from build123d import *

# Parameters (mm, degrees)
SKETCH_1_R          = 1.8
EXTRUDE_1_DEPTH     = 6.4
SKETCH_7_R          = 3
CUT_EXTRUDE_1_DEPTH = 3.2
SKETCH_8_R          = 4
SKETCH_8_R_2        = 1.8
EXTRUDE_2_DEPTH     = 5
SKETCH_9_R          = 5.65
SKETCH_9_R_2        = 4
CUT_EXTRUDE_2_DEPTH = 2


with BuildPart() as part:
    # Эскиз1 → Бобышка-Вытянуть1 (new body)
    with BuildSketch(Plane(origin=(0, 0, 0), x_dir=(1, 0, 0), z_dir=(0, 1, 0))):
        with BuildLine():
            Line((-10, 0), (-8.31553819, 3.436118058))
            ThreePointArc((-8.31553819, 3.436118058), (-1.40535605, 7.805603403), (5.613555936, 3.613003503))
            Line((5.613555936, 3.613003503), (7.5, 0))
            Line((7.5, 0), (5.613555936, -3.613003503))
            ThreePointArc((5.613555936, -3.613003503), (-1.40535605, -7.805603403), (-8.31553819, -3.436118058))
            Line((-8.31553819, -3.436118058), (-10, 0))
        make_face()
        Circle(SKETCH_1_R, mode=Mode.SUBTRACT)
    extrude(amount=EXTRUDE_1_DEPTH)

    # Эскиз7 → Вырез-Вытянуть1 (cut)
    with BuildSketch(Plane(origin=(0, 6.4, 0), x_dir=(1, 0, 0), z_dir=(0, 1, 0))):
        Circle(SKETCH_7_R)
    extrude(amount=-CUT_EXTRUDE_1_DEPTH, mode=Mode.SUBTRACT)

    # Эскиз8 → Бобышка-Вытянуть2 (add)
    with BuildSketch(Plane.XZ):
        Circle(SKETCH_8_R)
        Circle(SKETCH_8_R_2, mode=Mode.SUBTRACT)
    extrude(amount=EXTRUDE_2_DEPTH)

    # Эскиз9 → Вырез-Вытянуть2 (cut)
    with BuildSketch(Plane.XZ):
        Circle(SKETCH_9_R)
        Circle(SKETCH_9_R_2, mode=Mode.SUBTRACT)
    extrude(amount=-CUT_EXTRUDE_2_DEPTH, mode=Mode.SUBTRACT)


solid = part.part
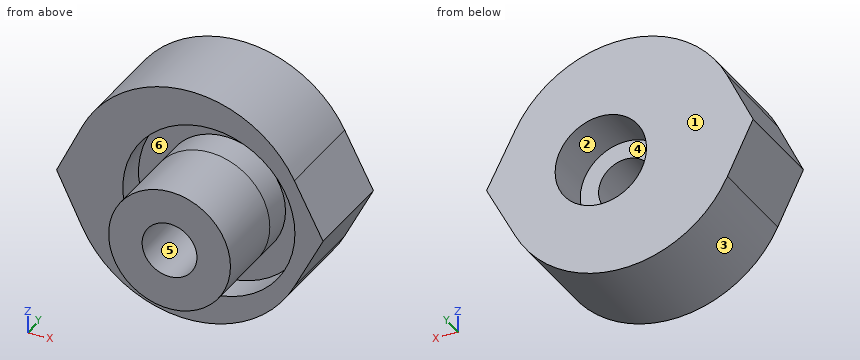
Geometry check sheet. Reference: the model listing, model coordinates, mm. Face numbers are marked on the shaded views. A direction names the side the tool comes from. Give positions to 0.01 mm unless a question says otherwise; leave off trailing zeros. Write each loop counter-clockwise with the first axis right and the second up, starting at its lowest first coordinate (ties: lowest second). Pieces come first, ordered by that corner, then holes. Notation, with made-up numbers: M -37.75,9 L -26.75,9 A31 ccw -26.75,48 Z; hole C -18.5,20.5 d2. An arc over 180 degrees is marked long. Answer as CSV lines item,"result". Start each with the question number.
Q1. Section check A-A, the plane y = 1.5. Record the cut outline in (x, z), then the cut area to 3 significant figures.
Q2. Go/stop test with flat-tipped pins: pin 1 (1 mm diameter, centred on y = 0, z = -3.5, fed in from -X); pin 2 (3 mm diameter, centred on x = 1, z = -0.5, fed in from +Y); pin 3 (1 mm diameter, centred on x = -7, y = 4.5, fed in from -Z). Record where each tip stops, or that it passes through.
Q3. Release check for a two-part mould opening along X. For the marked faces 1, 2, 3 and 4 record: pulls with the +X half, pulls with the -X half, needs draft (parallel to the pull), parting line crosses it, or undercut.
Q4. Tool access check on the marked faces 5 and 6. Record the directions out of +Z, -Z, +X, -X, +Y, -Y that give a thin tool (end or side, any length) a straight path to the whole face; none if there is none.
Q5. Section check B-B, the plane x = 0. Record the cut outline in (y, z).
Q6. Material ranges on L1, parallel to Z at x = 0, y = 0.5; L2, parallel to Y at x = -3.5, z = -3.25; L3, parallel to Y at x = -5.25, z = 4.25, recorded low to high.
Q7. Section check C-C, the plane y = 5.5. Record the cut outline in (x, z).
Q8. Section check D-D, the plane z = -4.5. Record the cut outline in (x, y).
Geometry says:
1,outline,"M -10,0 L -8.32,-3.44 A7.81 ccw 5.61,-3.61 L 7.5,0 L 5.61,3.61 A7.81 ccw -8.32,3.44 Z; C 0,0 d8; hole C 0,0 d11.3; hole C 0,0 d3.6"
1,area,"136 mm^2"
2,pin 1,"x = -8.53"
2,pin 2,"y = 3.2"
2,pin 3,"z = -5.83"
3,face 1,"needs draft"
3,face 2,"undercut"
3,face 3,"parting line crosses it"
3,face 4,"undercut"
4,face 5,"+Y, -Y"
4,face 6,"-Y"
5,outline,"M -5,-4 L 2,-4 L 2,-5.65 L 0,-5.65 L 0,-7.7 L 6.4,-7.7 L 6.4,-3 L 3.2,-3 L 3.2,-1.8 L -5,-1.8 Z; M -5,1.8 L 3.2,1.8 L 3.2,3 L 6.4,3 L 6.4,7.7 L 0,7.7 L 0,5.65 L 2,5.65 L 2,4 L -5,4 Z"
6,L1,"-7.7 to -5.65, -4 to -1.8, 1.8 to 4, 5.65 to 7.7"
6,L2,"2 to 6.4"
6,L3,"0 to 6.4"
7,outline,"M -10,0 L -8.32,-3.44 A7.81 ccw 5.61,-3.61 L 7.5,0 L 5.61,3.61 A7.81 ccw -8.32,3.44 Z; hole C 0,0 d6"
8,outline,"M -7.68,0 L -3.42,0 L -3.42,2 L 3.42,2 L 3.42,0 L 5.07,0 L 5.07,6.4 L -7.68,6.4 Z"
